The listing builds one solid part. Answer for the finished solid, in the listing's coordinates (mm). Face numbers are marked on the shaded views. Round coordinates to 2 decimals unless told otherwise and drop trailing zeros. Loops run counter-clockwise (first coordinate to the right, second up) from the corner with the lowest first, then second, coordinate; pieces in that order, holes last. Notation, with made-up numbers: M 38.25,89.5 L 84.25,89.5 A35 ccw 84.25,123.5 Z; hole C 48.25,31 d5. An arc over 180 degrees is marked long. Answer as a JSON object with one key per item and string values.
```python
from build123d import *

# Parameters (mm, degrees)
SKETCH_1_W          = 38
SKETCH_1_H          = 8
SKETCH_1_R          = 1.5
EXTRUDE_1_DEPTH     = 8
SKETCH_2_R          = 1.5
CUT_EXTRUDE_1_DEPTH = 9


with BuildPart() as part:
    # 草图1 → 凸台-拉伸1 (new body)
    with BuildSketch(Plane(origin=(0, 0, 0), x_dir=(1, 0, 0), z_dir=(0, 1, 0))):
        Rectangle(SKETCH_1_W, SKETCH_1_H)
        with Locations((-15, 0)):
            Circle(SKETCH_1_R, mode=Mode.SUBTRACT)
        with Locations((5, 0)):
            Circle(SKETCH_1_R, mode=Mode.SUBTRACT)
    extrude(amount=EXTRUDE_1_DEPTH)

    # 草图2 → 切除-拉伸1 (cut, through all)
    with BuildSketch(Plane.XY.offset(4)):
        with Locations((-5, 4)):
            Circle(SKETCH_2_R)
        with Locations((15, 4)):
            Circle(SKETCH_2_R)
    extrude(amount=-CUT_EXTRUDE_1_DEPTH, mode=Mode.SUBTRACT)


solid = part.part
```
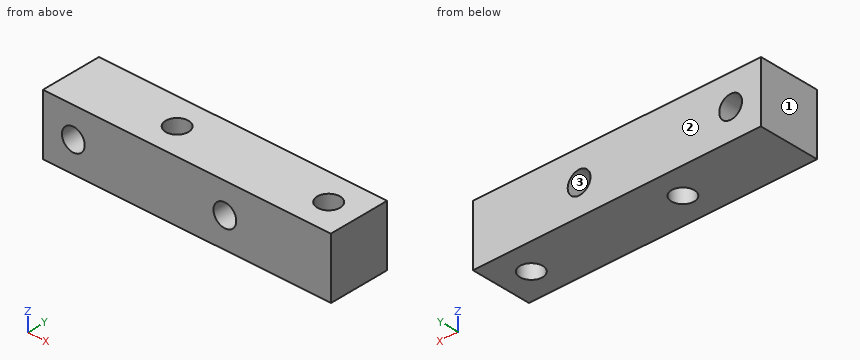
Item 1: Determine the mould class of the marked faces 1, 2 and 3 for opening direction X: released by +X, released by -X, zero draft, split by the parting line, or undercut.
Values follow:
{"face 1": "released by -X", "face 2": "zero draft", "face 3": "undercut"}
Item 2: A flat-ended cylindrical pin translates along its axis: P1, Ø2.5, axis at x = -5, y = 4, coming from the +Z side. Find the tip coordinate at first contact, or state that the pin passes through.
Values follow:
{"P1": "through"}
Item 3: The part is cut by section A-A (z = 0). Give the vertices of the cut face in (x, y), then the cut area to 3 significant figures.
Values follow:
{"outline": "M -19,0 L -16.5,0 L -16.5,8 L -19,8 Z; M -13.5,0 L 3.5,0 L 3.5,8 L -13.5,8 Z; M 6.5,0 L 19,0 L 19,8 L 6.5,8 Z; hole C -5,4 d3; hole C 15,4 d3", "area": "242 mm^2"}
Item 4: The part is cut by section D-D (z = -2). Give the vertices of the cut face in (x, y).
Values follow:
{"outline": "M -19,0 L 19,0 L 19,8 L -19,8 Z; hole C -5,4 d3; hole C 15,4 d3"}
Item 5: The part is cut by section B-B (x = 15). Give the vertices of the cut face in (y, z).
Values follow:
{"outline": "M 0,-4 L 2.5,-4 L 2.5,4 L 0,4 Z; M 5.5,-4 L 8,-4 L 8,4 L 5.5,4 Z"}
Item 6: The part is cut by section C-C (y = 1). Give the vertices of the cut face in (x, z), then the cut area to 3 significant figures.
Values follow:
{"outline": "M -19,-4 L 19,-4 L 19,4 L -19,4 Z; hole C -15,0 d3; hole C 5,0 d3", "area": "290 mm^2"}
Item 7: Straight lines are drawn through the part: line 1 (X direction, y = 2, z = 0); line 2 (Z direction, x = 5, y = 4.75); line 3 (X direction, y = 3.75, z = 0). For each, find the intervals that lie inside material, in ascending order.
Values follow:
{"line 1": "-19 to -16.5, -13.5 to 3.5, 6.5 to 19", "line 2": "-4 to -1.5, 1.5 to 4", "line 3": "-19 to -16.5, -13.5 to -6.48, -3.52 to 3.5, 6.5 to 13.52, 16.48 to 19"}
